The listing builds one solid part. Answer for the finished solid, in the listing's coordinates (mm). A direction names the side the tool comes from. Round coordinates to 2 decimals unless told otherwise and drop trailing zeros. Loops run counter-clockwise (first coordinate to the right, second up) from the corner with the lowest first, then second, coordinate; pieces in that order, holes last. Notation, with made-up numbers: (65, -12) - (81, -12) arc R10 cw to (81, 2) - close; hole circle Ø4 at (-10.75, 40.25). An arc over 180 degrees is marked (long way). Write item = value, one per line. Start each with the question number.
1) Straight lines are drawn through the part: line 1 along X through (y, z) = (2.3, 23); line 2 along X through (y, z) = (4.25, 23); line 3 along Y through (x, z) = (-17, 6). For each, find the intervals that lie inside material, in ascending order.
2) Section D-D, the plane x = -21 is taken. Determine the outline of the cut face in (y, z).
3) Section B-B, the plane z = 23 is taken. Determine the outline of the cut face in (x, y).
4) For a pull along Y with two mould halves and no side action, classify faces 6 (the flat face through (-25.04, 9.18, -6.01)), 7 (the cylindrical face through (15.64, 6.74, 0.37)), 8 (the cylindrical face through (0.42, 0.22, 0.11)), 9 (the flat face through (0, 3, 28)) as released by +Y, released by -Y, zero draft, split by the parting line, or undercut.
5) Section C-C, the plane z = 14 is taken. Determine the outline of the cut face in (x, y).
6) A tool of negligible diameter and unlimited length cuts with its end or side. For faces 1 (the flat face through (24.96, 9.18, -6.01)), 2 (the cylindrical face through (-11.923, 2.169, 10.245)), 3 (the flat face through (16.5, 3, 23)), 4 (the cylindrical face through (-14.272, 1.479, 21.265)), 5 (the flat face through (0.42, 19.48, -16.44)), from which of +Z, -Z, +X, -X, +Y, -Y can it reach the whole face along a straight path? Write none if from no direction.
7) Given pin 1 Ø4 at (x, z) = (14.5, -1) entering from +Y; pin 2 Ø1.8 at (x, z) = (15.5, 22.5) entering from +Y; pin 3 Ø2 at (x, y) = (-13, 19) entering from -Z; pin 4 Ø15 at (x, z) = (0, 14) entering from -Y, each flat-ended and moving along its own axis, determine where each tip first touches the part or whether it passes through.
8) Section A-A, the plane x = 4 is taken. Determine the outline of the cut face in (y, z), and give its area (3 significant figures).
from build123d import *

# Parameters (mm, degrees)
SALIENTE_EXTRUIR1_DEPTH      = 30
SALIENTE_EXTRUIR1_DEPTH_BACK = 30
CROQUIS3_R                   = 1.75
CORTAR_EXTRUIR1_DEPTH        = 4.242641
CROQUIS4_R                   = 3
CORTAR_EXTRUIR2_DEPTH        = 2
CROQUIS5_R                   = 10
CROQUIS5_R_2                 = 1.75
CORTAR_EXTRUIR3_DEPTH        = 6
CROQUIS5_4_R                 = 12.5
CROQUIS5_4_R_2               = 10
CORTAR_EXTRUIR4_DEPTH        = 4.4
REDONDEO1_R                  = 10
REDONDEO2_R                  = 3
REDONDEO3_R                  = 10
CROQUIS6_R                   = 3
CORTAR_EXTRUIR5_DEPTH        = 3


with BuildPart() as part:
    # Croquis2 → Saliente-Extruir1 (new body, two sides)
    with BuildSketch(Plane(origin=(0, 0, 0), x_dir=(0, 0, -1), z_dir=(1, 0, 0))) as saliente_extruir1_sk:
        Polygon((0, 0), (-28, 0), (-28, 6), (0, 6), (14.960512242, 20.960512242), (17.960512242, 17.960512242), align=None)
    extrude(amount=SALIENTE_EXTRUIR1_DEPTH)
    extrude(saliente_extruir1_sk.sketch, amount=-SALIENTE_EXTRUIR1_DEPTH_BACK)

    # Croquis3 → Cortar-Extruir1 (cut)
    with BuildSketch(Plane(origin=(0, 0, 0), x_dir=(-1, 0, 0), z_dir=(0, -0.707106781, -0.707106781))):
        with Locations((-25, 12.7)):
            Circle(CROQUIS3_R)
        with Locations((25, 12.7)):
            Circle(CROQUIS3_R)
    extrude(amount=-CORTAR_EXTRUIR1_DEPTH, mode=Mode.SUBTRACT)

    # Croquis4 → Cortar-Extruir2 (cut)
    with BuildSketch(Plane(origin=(0, 3, 3), x_dir=(1, 0, 0), z_dir=(0, 0.707106781, 0.707106781))):
        with Locations((-25, 12.7)):
            Circle(CROQUIS4_R)
        with Locations((25, 12.7)):
            Circle(CROQUIS4_R)
    extrude(amount=-CORTAR_EXTRUIR2_DEPTH, mode=Mode.SUBTRACT)

    # Croquis5 → Cortar-Extruir3 (cut)
    with BuildSketch(Plane(origin=(0, 0, 0), x_dir=(-1, 0, 0), z_dir=(0, -1, 0))):
        with Locations((0, -14)):
            Circle(CROQUIS5_R)
        with Locations((14.5, -23)):
            Circle(CROQUIS5_R_2)
        with Locations((-14.5, -23)):
            Circle(CROQUIS5_R_2)
        with BuildLine():
            ThreePointArc((-19.082136833, -25.001005257), (-17.238153914, -27.1836005), (-14.5, -28))
            Line((-14.5, -28), (-30, -28))
            Line((-30, -28), (-30, 0))
            Line((-30, 0), (-19.082136833, -25.001005257))
        make_face()
        with BuildLine():
            Line((30, 0), (19.082136833, -25.001005257))
            ThreePointArc((19.082136833, -25.001005257), (17.238153914, -27.1836005), (14.5, -28))
            Line((14.5, -28), (30, -28))
            Line((30, -28), (30, 0))
        make_face()
    extrude(amount=-CORTAR_EXTRUIR3_DEPTH, mode=Mode.SUBTRACT)

    # Croquis5<4> → Cortar-Extruir4 (cut)
    with BuildSketch(Plane(origin=(0, 0, 0), x_dir=(-1, 0, 0), z_dir=(0, -1, 0))):
        with Locations((0, -14)):
            Circle(CROQUIS5_4_R)
        with Locations((0, -14)):
            Circle(CROQUIS5_4_R_2, mode=Mode.SUBTRACT)
    extrude(amount=-CORTAR_EXTRUIR4_DEPTH, mode=Mode.SUBTRACT)

    # Redondeo1
    redondeo1_edges = [part.edges().sort_by_distance(p)[0] for p in [
        (0, 6, 0),
    ]]
    fillet(redondeo1_edges, radius=REDONDEO1_R)

    # Redondeo2
    redondeo2_edges = [part.edges().sort_by_distance(p)[0] for p in [
        (0, 0, 0),
    ]]
    fillet(redondeo2_edges, radius=REDONDEO2_R)

    # Redondeo3
    redondeo3_edges = [part.edges().sort_by_distance(p)[0] for p in [
        (-30, 3.583831813, 0),
        (30, 3.583831813, 0),
    ]]
    fillet(redondeo3_edges, radius=REDONDEO3_R)

    # Croquis6 → Cortar-Extruir5 (cut)
    with BuildSketch(Plane(origin=(0, 6, 0), x_dir=(1, 0, 0), z_dir=(0, 1, 0))):
        with Locations((14.5, -23)):
            Circle(CROQUIS6_R)
        with Locations((-14.5, -23)):
            Circle(CROQUIS6_R)
    extrude(amount=-CORTAR_EXTRUIR5_DEPTH, mode=Mode.SUBTRACT)


solid = part.part
Geometry check:
q1.line_1 = -19.96 to -16.25, -12.75 to -8.67, 8.67 to 12.75, 16.25 to 19.96
q1.line_2 = -19.96 to -17.5, -11.5 to -8.67, 8.67 to 11.5, 17.5 to 19.96
q1.line_3 = 0 to 6
q2.outline = (0, 1.24) arc R3 ccw to (0.88, -0.88) - (17.96, -17.96) - (20.96, -14.96) - (8.93, -2.93) arc R10 cw to (6, 4.14) - (6, 20.61) - (0, 20.61) - close
q3.outline = (-19.96, 0) - (-16.25, 0) - (-16.25, 3) - (-17.5, 3) - (-17.5, 6) - (-19.96, 6) - close; (-12.75, 0) - (-8.67, 0) - (-8.67, 4.4) - (-4.36, 4.4) - (-4.36, 6) - (-11.5, 6) - (-11.5, 3) - (-12.75, 3) - close; (4.36, 4.4) - (8.67, 4.4) - (8.67, 0) - (12.75, 0) - (12.75, 3) - (11.5, 3) - (11.5, 6) - (4.36, 6) - close; (16.25, 0) - (19.96, 0) - (19.96, 6) - (17.5, 6) - (17.5, 3) - (16.25, 3) - close
q4.face_6 = undercut
q4.face_7 = released by +Y
q4.face_8 = released by -Y
q4.face_9 = zero draft
q5.outline = (-23.89, 0) - (-12.5, 0) - (-12.5, 4.4) - (-10, 4.4) - (-10, 6) - (-23.89, 6) - close; (10, 4.4) - (12.5, 4.4) - (12.5, 0) - (23.89, 0) - (23.89, 6) - (10, 6) - close
q6.face_1 = none
q6.face_2 = -Y
q6.face_3 = +Y
q6.face_4 = +Y, -Y
q6.face_5 = -Z, +X, -X, +Y
q7.pin_1 = 9
q7.pin_2 = 3
q7.pin_3 = -17.92
q7.pin_4 = through
q8.outline = (0, 1.24) arc R3 ccw to (0.88, -0.88) - (17.96, -17.96) - (20.96, -14.96) - (8.93, -2.93) arc R10 cw to (6, 4.14) - (6, 4.83) - (4.4, 4.83) - (4.4, 2.16) - (0, 2.16) - close; (0, 25.84) - (4.4, 25.84) - (4.4, 23.17) - (6, 23.17) - (6, 28) - (0, 28) - close
q8.area = 135 mm2
